Part model, mm, in its own coordinate system. Face numbers are marked on the shaded views. A direction names the side the tool comes from. Round coordinates to 2 decimals unless told otherwise and drop trailing zeros. Write each loop counter-clockwise with the first axis right and the second up, starting at its lowest first coordinate (ties: lowest second). Pieces come first, ordered by that corner, then holes. Notation, with made-up numbers: M 43.25,50 L 85.25,50 A32 ccw 85.25,89 Z; hole C -0.75,88 d9. An arc over 180 degrees is marked long. One line per question, with ' | ' between items. Start each with the question number.
1) Saw through at B-B (x = -16). List the corners of the cut face in (y, z), plus the area to 3 significant figures.
2) Saw through at C-C (y = 6). List the corners of the cut face in (x, z).
3) Wall check: probe 1 along Y at (x, z) = (16, 3); probe 2 along X at (y, z) = (4.5, 0.75); probe 3 along X at (y, z) = (5.75, 0.5). Give the ranges that are in metal, low to high. Write a range as [from, to].
4) Saw through at D-D (z = 0.5). List the corners of the cut face in (x, y), plus the area to 3 significant figures.
5) Tool access for the marked faces 4 and 5: list every direction of +Z, -Z, +X, -X, +Y, -Y with a clear straight run to the whole face (end or side of a thin tool).
6) Drop flat-ended pins along their axis: pin 1 Ø1.6 at (y, z) = (0.5, 5) entering from -X; pin 2 Ø1 at (y, z) = (0.5, 5.5) entering from +X; pin 3 Ø0.6 at (x, y) = (5.5, 1) entering from +Z; pin 4 Ø1.5 at (x, z) = (2, 4.5) entering from +Y (1 decimal). Give the stop position or say it passes through.
7) Mould opens along X. For the marked faces 1, 2 and 3 say: pulls with the +X half, pulls with the -X half, needs draft (parallel to the pull), parting line crosses it, or undercut.
8) Saw through at A-A (z = 6.5). List the corners of the cut face in (x, y).
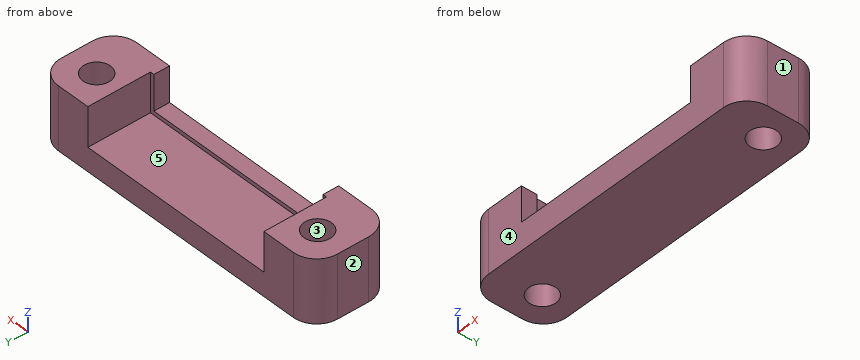
```python
from build123d import *

# Parameters (mm, degrees)
SKETCH1_R           = 1.75
BOSS_EXTRUDE1_DEPTH = 8
SKETCH2_W           = 25.5
SKETCH2_H           = 8
CUT_EXTRUDE1_DEPTH  = 5
SKETCH3_W           = 24.5
SKETCH3_H           = 4.5
CUT_EXTRUDE2_DEPTH  = 3


with BuildPart() as part:
    # Sketch1 → Boss-Extrude1 (new body)
    with BuildSketch(Plane.XY):
        with BuildLine():
            Line((-17, 10), (17, 10))
            ThreePointArc((17, 10), (19.121320344, 9.121320344), (20, 7))
            Line((20, 7), (20, 3))
            ThreePointArc((20, 3), (19.121320344, 0.878679656), (17, 0))
            Line((17, 0), (-17, 0))
            ThreePointArc((-17, 0), (-19.121320344, 0.878679656), (-20, 3))
            Line((-20, 3), (-20, 7))
            ThreePointArc((-20, 7), (-19.121320344, 9.121320344), (-17, 10))
        make_face()
        with Locations((-16, 6)):
            Circle(SKETCH1_R, mode=Mode.SUBTRACT)
        with Locations((16, 6)):
            Circle(SKETCH1_R, mode=Mode.SUBTRACT)
    extrude(amount=BOSS_EXTRUDE1_DEPTH)

    # Sketch2 → Cut-Extrude1 (cut)
    with BuildSketch(Plane.XY.offset(8)):
        with Locations((0, 6)):
            Rectangle(SKETCH2_W, SKETCH2_H)
    extrude(amount=-CUT_EXTRUDE1_DEPTH, mode=Mode.SUBTRACT)

    # Sketch3 → Cut-Extrude2 (cut, through all)
    with BuildSketch(Plane(origin=(0, 2, 0), x_dir=(1, 0, 0), z_dir=(0, 1, 0))):
        with Locations((0, -5.75)):
            Rectangle(SKETCH3_W, SKETCH3_H)
    extrude(amount=-CUT_EXTRUDE2_DEPTH, mode=Mode.SUBTRACT)


solid = part.part
```
Answer key:
1) outline: M 0,0 L 4.25,0 L 4.25,8 L 0,8 Z; M 7.75,0 L 10,0 L 10,8 L 7.75,8 Z | area: 52.0 mm2
2) outline: M -20,0 L -17.75,0 L -17.75,8 L -20,8 Z; M -14.25,0 L 14.25,0 L 14.25,8 L 12.75,8 L 12.75,3 L -12.75,3 L -12.75,8 L -14.25,8 Z; M 17.75,0 L 20,0 L 20,8 L 17.75,8 Z
3) probe 1: y = [0, 4.25], [7.75, 10] | probe 2: x = [-20, -16.9], [-15.1, 15.1], [16.9, 20] | probe 3: x = [-20, -17.73], [-14.27, 14.27], [17.73, 20]
4) outline: M -20,3 A3 ccw -17,0 L 17,0 A3 ccw 20,3 L 20,7 A3 ccw 17,10 L -17,10 A3 ccw -20,7 Z; hole C -16,6 d3.5; hole C 16,6 d3.5 | area: 373 mm2
5) face 4: +Z, -Z, +X, -X, -Y | face 5: +Z, +Y
6) pin 1: stops at x = -19.47 | pin 2: stops at x = 19.24 | pin 3: stops at z = 3.5 | pin 4: passes through
7) face 1: pulls with the +X half | face 2: pulls with the -X half | face 3: undercut
8) outline: M -20,3 A3 ccw -17,0 L -12.25,0 L -12.25,2 L -12.75,2 L -12.75,10 L -17,10 A3 ccw -20,7 Z; M 12.25,0 L 17,0 A3 ccw 20,3 L 20,7 A3 ccw 17,10 L 12.75,10 L 12.75,2 L 12.25,2 Z; hole C -16,6 d3.5; hole C 16,6 d3.5
